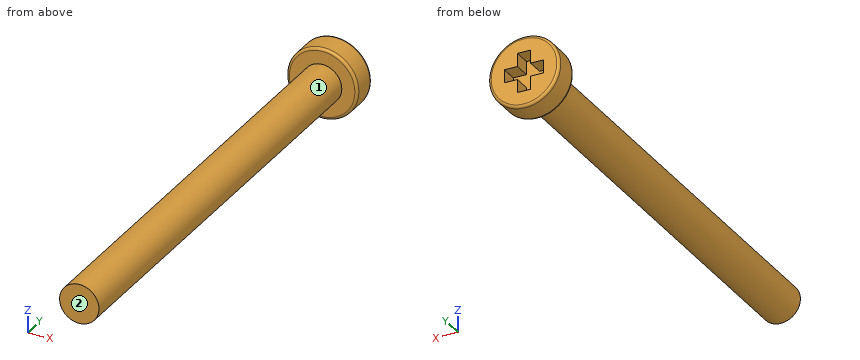
```python
from build123d import *

# Parameters (mm, degrees)
FILLET_R     = 0.2
POCKET_DEPTH = 1.3


with BuildPart() as part:
    # Sketch → Revolution (revolve)
    with BuildSketch(Plane.XY):
        Polygon((0, 0), (0, 37), (2.7, 37), (2.7, 35), (1.5, 35), (1.5, 0), align=None)
    revolve(axis=Axis((0, 0, 0), (0, 1, 0)))

    # Fillet
    fillet_edges = [part.edges().sort_by_distance(p)[0] for p in [
        (-2.7, 35, 0),
        (-2.7, 37, 0),
    ]]
    fillet(fillet_edges, radius=FILLET_R)

    # Sketch001 (on Face1 of Fillet) → Pocket (cut)
    with BuildSketch(Plane(origin=(0, 37, 0), x_dir=(-1, 0, 0), z_dir=(0, 1, 0))):
        Polygon((0.5, 1.5), (0.5, 0.5), (1.5, 0.5), (1.5, -0.5), (0.5, -0.5), (0.5, -1.5), (-0.5, -1.5), (-0.5, -0.5), (-1.5, -0.5), (-1.5, 0.5), (-0.5, 0.5), (-0.5, 1.5), align=None)
    extrude(amount=-POCKET_DEPTH, mode=Mode.SUBTRACT)


solid = part.part
```
Check sheet for the modelled part. Datum: model origin and axes. Units: mm. Face numbers are marked on the shaded views. A direction names the side the tool comes from. Give positions to 0.01 mm unless a question says otherwise; leave off trailing zeros. Order: outer loops, then holes, each group sorted by start corner. A loop starts at its lowest first (then second) coordinate and runs counter-clockwise, first axis right, second up. Notation, with made-up numbers: M 2,18.25 L 9,18.25 A29 ccw 9,53.25 Z; hole C 19.5,51 d5. An arc over 180 degrees is marked long. Answer in a Markdown table with one row per item. Add a question column.
Q1. Access from +Z, -Z, +X, -X, +Y, -Y to the whole of each face (thin tool, end or side, straight path). Record for the marked faces 1 and 2.
Q2. Sectioned sample at B-B, the plane z = 0. Record the boundary of the cut face in (x, y), and give its area (3 significant figures).
Q3. Sectioned sample at C-C, the plane y = 22.5. Record the boundary of the cut face in (x, z).
Q4. Gauge pin test, flat ends, axial feed: pin 1 Ø0.8 at (x, y) = (-1, 36.5) entering from +Z; pin 2 Ø1.1 at (x, y) = (-1, 36.5) entering from -Z; pin 3 Ø2 at (y, z) = (31.5, 1.5) entering from +X. Record the tip position at first contact, or that the pin passes through.
Q5. Thickness scan on L1, parallel to Y at x = -1.3, z = -1.6; L2, parallel to Y at x = 0.2, z = 1.1; L3, parallel to Z at x = 0.1, y = 6. Record the ranges inside material, lowest first.
Q6. Sectioned sample at A-A, the plane x = 0. Record the boundary of the cut face in (y, z), and give its area (3 significant figures).
Verdict:
| question | item | result |
|---|---|---|
| 1 | face 1 | -Y |
| 1 | face 2 | +Z, -Z, +X, -X, -Y |
| 2 | outline | M -2.7,35.2 A0.2 ccw -2.5,35 L -1.5,35 L -1.5,0 L 1.5,0 L 1.5,35 L 2.5,35 A0.2 ccw 2.7,35.2 L 2.7,36.8 A0.2 ccw 2.5,37 L 1.5,37 L 1.5,35.7 L -1.5,35.7 L -1.5,37 L -2.5,37 A0.2 ccw -2.7,36.8 Z |
| 2 | area | 112 mm² |
| 3 | outline | C 0,0 d3 |
| 4 | pin 1 | z = 2.63 |
| 4 | pin 2 | z = -2.66 |
| 4 | pin 3 | x = 1.41 |
| 5 | L1 | 35 to 37 |
| 5 | L2 | 0 to 35.7 |
| 5 | L3 | -1.5 to 1.5 |
| 6 | outline | M 0,-1.5 L 35,-1.5 L 35,-2.5 A0.2 ccw 35.2,-2.7 L 36.8,-2.7 A0.2 ccw 37,-2.5 L 37,-1.5 L 35.7,-1.5 L 35.7,1.5 L 37,1.5 L 37,2.5 A0.2 ccw 36.8,2.7 L 35.2,2.7 A0.2 ccw 35,2.5 L 35,1.5 L 0,1.5 Z |
| 6 | area | 112 mm² |
